Check sheet for the modelled part. Datum: model origin and axes. Units: mm. Round coordinates to 2 decimals unless told otherwise and drop trailing zeros. Loops run counter-clockwise (first coordinate to the right, second up) from the corner with the lowest first, then second, coordinate; pieces in that order, holes last. Notation, with made-up numbers: (84, -39.75) - (93, -39.75) arc R25 cw to (93, -5.75) - close; hole circle Ø1 at (15, 50). An arc over 180 degrees is marked (long way). Put each result on its own line as item: value.
```python
from build123d import *

# Parameters (mm, degrees)
ESQUISSE1_R        = 2.25
BOSS_EXTRU_1_DEPTH = 2


with BuildPart() as part:
    # Esquisse1 → Boss.-Extru.1 (new body)
    with BuildSketch(Plane.XY):
        with BuildLine():
            Line((0, 6.5), (50, 6.5))
            ThreePointArc((50, 6.5), (53.535533906, 5.035533906), (55, 1.5))
            Line((55, 1.5), (55, -1.5))
            ThreePointArc((55, -1.5), (53.535533906, -5.035533906), (50, -6.5))
            Line((50, -6.5), (0, -6.5))
            ThreePointArc((0, -6.5), (-3.535533906, -5.035533906), (-5, -1.5))
            Line((-5, -1.5), (-5, 1.5))
            ThreePointArc((-5, 1.5), (-3.535533906, 5.035533906), (0, 6.5))
        make_face()
        Circle(ESQUISSE1_R, mode=Mode.SUBTRACT)
        with Locations((50, 0)):
            Circle(ESQUISSE1_R, mode=Mode.SUBTRACT)
    extrude(amount=BOSS_EXTRU_1_DEPTH)


solid = part.part
```
Item 1: Section check D-D on y = 5.5. Enter the section's corners in (x, z).
Filled sheet:
outline: (-3, 0) - (53, 0) - (53, 2) - (-3, 2) - close
Item 2: Release check for a two-part mould opening along X. For faces 1 (the cylindrical face through (47.752, 0.099, 0.986)), 2 (the cylindrical face through (53.5, 5.07, 0.99)), 3 (the flat face through (25, 0, 0)) record: +X half, -X half, draft (parallel to the pull), parting line (faces both ways), or undercut.
Filled sheet:
face 1: undercut
face 2: +X half
face 3: draft
Item 3: Go/stop test with a flat-tipped pin: pin 1 (1 mm diameter, centred on x = 45.5, y = -1.5, fed in from -Z). Record where the tip stops, or that it passes through.
Filled sheet:
pin 1: z = 0
Item 4: Section check B-B on z = 0.45. Enter the section's corners in (x, y).
Filled sheet:
outline: (-5, -1.5) arc R5 ccw to (0, -6.5) - (50, -6.5) arc R5 ccw to (55, -1.5) - (55, 1.5) arc R5 ccw to (50, 6.5) - (0, 6.5) arc R5 ccw to (-5, 1.5) - close; hole circle Ø4.5 at (0, 0); hole circle Ø4.5 at (50, 0)
Item 5: Section check A-A on y = 0. Enter the section's corners in (x, z), then the cut area to 3 significant figures.
Filled sheet:
outline: (-5, 0) - (-2.25, 0) - (-2.25, 2) - (-5, 2) - close; (2.25, 0) - (47.75, 0) - (47.75, 2) - (2.25, 2) - close; (52.25, 0) - (55, 0) - (55, 2) - (52.25, 2) - close
area: 102 mm²
Item 6: Thickness scan on line 1 (X direction, y = -0.5, z = 1); line 2 (X direction, y = -1.75, z = 1.75); line 3 (X direction, y = -3.75, z = 0.5). Record the ranges inside material, lowest first. Write a range as from..to.
Filled sheet:
line 1: -5..-2.19, 2.19..47.81, 52.19..55
line 2: -4.99..-1.41, 1.41..48.59, 51.41..54.99
line 3: -4.47..54.47
Item 7: Section check C-C on y = -4.5. Enter the section's corners in (x, z), then the cut area to 3 significant figures.
Filled sheet:
outline: (-4, 0) - (54, 0) - (54, 2) - (-4, 2) - close
area: 116 mm²
